Can you work these out from the drawing? Everything is in mm from the part's minimum corner. A direction names the side the tool comes from. Round coordinates to 2 decimals unless told otherwise and drop trailing zeros. Order: outer loops, then holes, each group sorted by start corner. A loop starts at its lowest first (then second) coordinate and runs counter-clockwise, first axis right, second up. Notation, with made-up numbers: (76.5, 5) -> (99.5, 5) arc R16 cw to (99.5, 13) -> close; hole circle Ø5 at (-39.5, 51). An arc over 180 degrees is marked (long way). One line per item, written item: value.
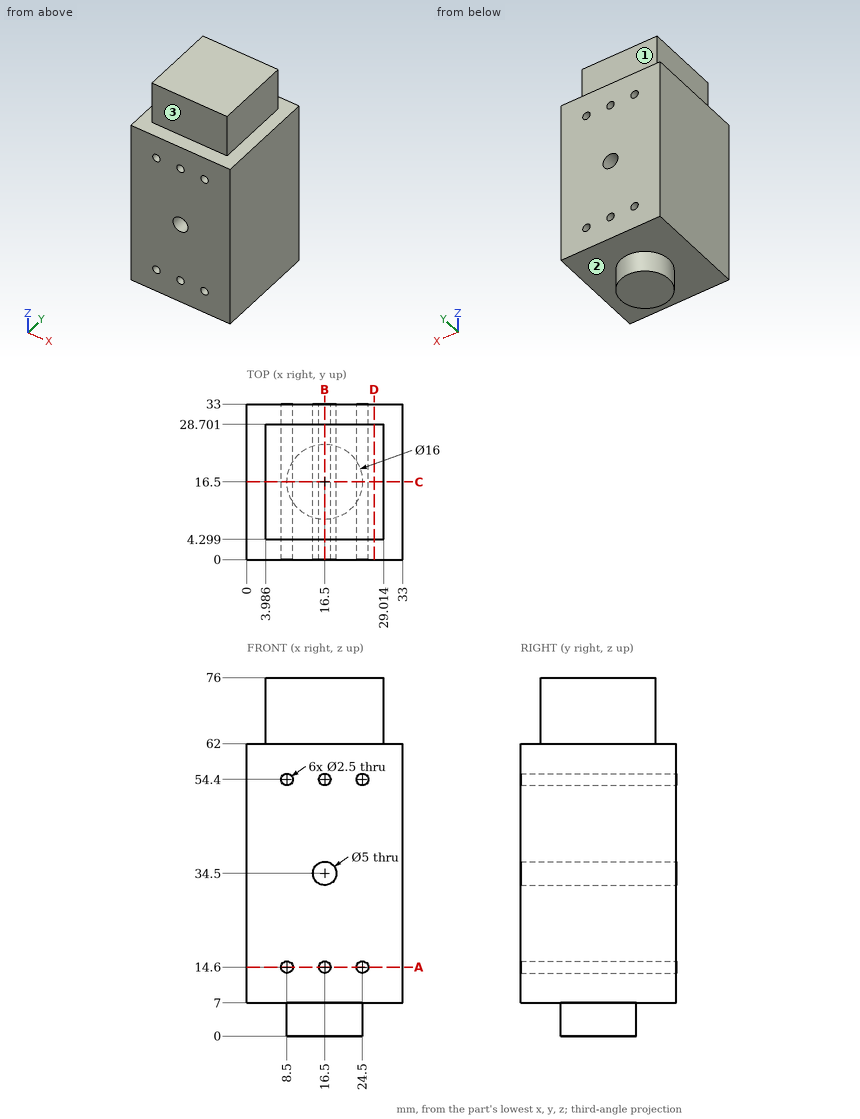
Q1. On a 3-axis mill with a long thin cutter (end or side, diameter ignored), from which of +Z, -Z, +X, -X, +Y, -Y can I reach the whole of each face in a straight line? I mean the marked faces 1, 2 and 3. Say none if no direction works.
Answers below:
face 1: +Z, +X, -X, +Y
face 2: -Z
face 3: +Z, +X, -X, -Y
Q2. I want a section at A-A on z = 14.6. List the corners of the cut face in (x, y) for me.
Answers below:
outline: (0, 0) -> (7.25, 0) -> (7.25, 33) -> (0, 33) -> close; (9.75, 0) -> (15.25, 0) -> (15.25, 33) -> (9.75, 33) -> close; (17.75, 0) -> (23.25, 0) -> (23.25, 33) -> (17.75, 33) -> close; (25.75, 0) -> (33, 0) -> (33, 33) -> (25.75, 33) -> close
Q3. Please list where these lines run through material, in increasing order: line 1 along Z through (x, y) = (16.5, 21); line 2 along Z through (x, y) = (8.5, 19.5); line 3 along X through (y, z) = (7, 14).
Answers below:
line 1: 0 to 13.35, 15.85 to 32, 37 to 53.15, 55.65 to 76
line 2: 7 to 13.35, 15.85 to 53.15, 55.65 to 76
line 3: 0 to 7.4, 9.6 to 15.4, 17.6 to 23.4, 25.6 to 33
Q4. I want a section at B-B on x = 16.5. List the corners of the cut face in (y, z) for me, plus the area to 3 significant figures.
Answers below:
outline: (0, 7) -> (8.5, 7) -> (8.5, 0) -> (24.5, 0) -> (24.5, 7) -> (33, 7) -> (33, 13.35) -> (0, 13.35) -> close; (0, 15.85) -> (33, 15.85) -> (33, 32) -> (0, 32) -> close; (0, 37) -> (33, 37) -> (33, 53.15) -> (0, 53.15) -> close; (0, 55.65) -> (33, 55.65) -> (33, 62) -> (28.7, 62) -> (28.7, 76) -> (4.3, 76) -> (4.3, 62) -> (0, 62) -> close
area: 1,940 mm^2
Q5. Will these pins go through, and if not, where does the flat tip stop? pin 1 Ø1.5 at (x, y) = (9.5, 27) entering from -Z; pin 2 Ø4 at (y, z) = (18, 70) entering from +X; pin 3 Ø15.5 at (y, z) = (15, 70.5) entering from -X.
Answers below:
pin 1: z = 7
pin 2: x = 29.01
pin 3: x = 3.99
Q6. I want a section at D-D on x = 27. List the corners of the cut face in (y, z) for me, plus the area to 3 significant figures.
Answers below:
outline: (0, 7) -> (33, 7) -> (33, 62) -> (28.7, 62) -> (28.7, 76) -> (4.3, 76) -> (4.3, 62) -> (0, 62) -> close
area: 2,160 mm^2
Q7. I want a section at C-C on y = 16.5. List the corners of the cut face in (x, z) for me.
Answers below:
outline: (0, 7) -> (8.5, 7) -> (8.5, 0) -> (24.5, 0) -> (24.5, 7) -> (33, 7) -> (33, 62) -> (29.01, 62) -> (29.01, 76) -> (3.99, 76) -> (3.99, 62) -> (0, 62) -> close; hole circle Ø2.5 at (8.5, 14.6); hole circle Ø2.5 at (8.5, 54.4); hole circle Ø5 at (16.5, 34.5); hole circle Ø2.5 at (16.5, 14.6); hole circle Ø2.5 at (16.5, 54.4); hole circle Ø2.5 at (24.5, 14.6); hole circle Ø2.5 at (24.5, 54.4)
